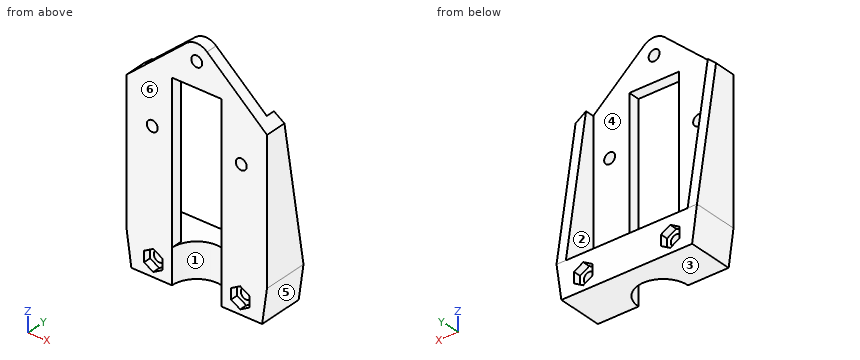
```python
from build123d import *

# Parameters (mm, degrees)
BOSS_EXTRUDE3_DEPTH              = 14.5
SKETCH8_R                        = 7.935
CUT_EXTRUDE3_DEPTH               = 88
CUT_EXTRUDE9_DEPTH               = 2.4
F_39_0_13779528_DIAMETER_HOLE1_D = 3.500000112
CUT_EXTRUDE10_DEPTH              = 22.4
CUT_EXTRUDE11_DEPTH              = 2.4
BOSS_EXTRUDE7_DEPTH              = 3.625
F_39_0_13779528_DIAMETER_HOLE2_D = 3.500000112
BOSS_EXTRUDE10_DEPTH             = 3
BOSS_EXTRUDE11_DEPTH             = 3
CUT_EXTRUDE14_DEPTH              = 13
CUT_EXTRUDE15_DEPTH              = 13
FILLET1_R                        = 5


with BuildPart() as part:
    # Sketch6 → Boss-Extrude3 (new body)
    with BuildSketch(Plane(origin=(0, 0, 0), x_dir=(1, 0, 0), z_dir=(0, 1, 0))):
        Polygon((-16.836914056, 5.783353512), (13.163085944, 5.783353512), (20.663085944, -47.581919406), (-24.336914056, -47.581919406), align=None)
    extrude(amount=BOSS_EXTRUDE3_DEPTH)

    # Sketch8 → Cut-Extrude3 (cut)
    with BuildSketch(Plane.XY.offset(47.581919406)):
        with Locations((-1.836914056, 0)):
            Circle(SKETCH8_R)
    extrude(amount=-CUT_EXTRUDE3_DEPTH, mode=Mode.SUBTRACT)

    # Sketch18 → Cut-Extrude9 (cut)
    with BuildSketch(Plane(origin=(0, 14.5, 0), x_dir=(1, 0, 0), z_dir=(0, 1, 0))):
        Polygon((-15.771819769, -44.868285994), (-12.821819769, -43.1651027), (-12.821819769, -39.758736112), (-15.771819769, -38.055552818), (-18.721819769, -39.758736112), (-18.721819769, -43.1651027), align=None)
        Polygon((12.097991657, -44.868285994), (15.047991657, -43.1651027), (15.047991657, -39.758736112), (12.097991657, -38.055552818), (9.147991657, -39.758736112), (9.147991657, -43.1651027), align=None)
        Polygon((11.389331688, -26.016021021), (14.389331688, -24.283970214), (14.389331688, -20.819868599), (11.389331688, -19.087817791), (8.389331688, -20.819868599), (8.389331688, -24.283970214), align=None)
        Polygon((-15.0631598, -26.016021021), (-12.0631598, -24.283970214), (-12.0631598, -20.819868599), (-15.0631598, -19.087817791), (-18.0631598, -20.819868599), (-18.0631598, -24.283970214), align=None)
    extrude(amount=-CUT_EXTRUDE9_DEPTH, mode=Mode.SUBTRACT)

    # #39 (0.13779528) Diameter Hole1 (through all)
    with Locations(Plane(origin=(-15.0631598, 14.5, 22.551919406), x_dir=(0, 0, 1), z_dir=(0, 1, 0))):
        with Locations((0, 0), (0, 26.452491488), (18.91, -0.708659969), (18.91, 27.161151457)):
            Hole(F_39_0_13779528_DIAMETER_HOLE1_D / 2)

    # Sketch22 → Cut-Extrude10 (cut)
    with BuildSketch(Plane(origin=(0, 14.5, 0), x_dir=(1, 0, 0), z_dir=(0, 1, 0))):
        Polygon((-22.781301734, -36.51316259), (19.107473622, -36.51316259), (13.163085944, 5.783353512), (-16.836914056, 5.783353512), align=None)
    extrude(amount=-CUT_EXTRUDE10_DEPTH, mode=Mode.SUBTRACT)

    # Sketch24 → Cut-Extrude11 (cut)
    with BuildSketch(Plane.XZ):
        Polygon((-15.771819769, 38.055552818), (-12.821819769, 39.758736112), (-12.821819769, 43.1651027), (-15.771819769, 44.868285994), (-18.721819769, 43.1651027), (-18.721819769, 39.758736112), align=None)
        Polygon((12.097991657, 38.055552818), (15.047991657, 39.758736112), (15.047991657, 43.1651027), (12.097991657, 44.868285994), (9.147991657, 43.1651027), (9.147991657, 39.758736112), align=None)
    extrude(amount=-CUT_EXTRUDE11_DEPTH, mode=Mode.SUBTRACT)

    # Sketch27 → Boss-Extrude7 (add)
    with BuildSketch(Plane(origin=(0, 0, 0), x_dir=(1, 0, 0), z_dir=(0, 1, 0))):
        Polygon((6.098085944, -47.581919406), (20.663085944, -47.581919406), (20.663085944, -112.581919406), (-9.771914056, -112.581919406), (-24.336914056, -112.581919406), (-24.336914056, -47.581919406), (-9.771914056, -47.581919406), (-9.771914056, -97.661919406), (6.098085944, -97.661919406), align=None)
    extrude(amount=BOSS_EXTRUDE7_DEPTH)

    # #39 (0.13779528) Diameter Hole2 (through all)
    with Locations(Plane(origin=(-16.086914056, 3.625, 80.900195398), x_dir=(0, 0, 1), z_dir=(0, 1, 0))):
        with Locations((0, 0), (24.681724008, 14.25), (0, 28.5)):
            Hole(F_39_0_13779528_DIAMETER_HOLE2_D / 2)

    # Sketch39 → Boss-Extrude10 (add)
    with BuildSketch(Plane(origin=(20.663085944, 0, 0), x_dir=(0, 0, -1), z_dir=(1, 0, 0))):
        Polygon((-47.581919406, 14.5), (-112.581919406, 3.625), (-47.581919406, 3.625), align=None)
    extrude(amount=-BOSS_EXTRUDE10_DEPTH)

    # Sketch40 → Boss-Extrude11 (add)
    with BuildSketch(Plane.ZY.offset(24.336914056)):
        Polygon((47.581919406, 14.5), (112.581919406, 3.625), (47.581919406, 3.625), align=None)
    extrude(amount=-BOSS_EXTRUDE11_DEPTH)

    # Sketch43 → Cut-Extrude14 (cut)
    with BuildSketch(Plane.XZ):
        Polygon((-1.836914056, 112.581919406), (-24.336914056, 112.581919406), (-24.336914056, 92.810231668), align=None)
    extrude(amount=-CUT_EXTRUDE14_DEPTH, mode=Mode.SUBTRACT)

    # Sketch44 → Cut-Extrude15 (cut)
    with BuildSketch(Plane.XZ):
        Polygon((20.663085944, 92.810231668), (20.663085944, 112.581919406), (-1.836914056, 112.581919406), align=None)
    extrude(amount=-CUT_EXTRUDE15_DEPTH, mode=Mode.SUBTRACT)

    # Fillet1
    fillet1_edges = [part.edges().sort_by_distance(p)[0] for p in [
        (-1.836914056, 1.8125, 112.581919406),
    ]]
    fillet(fillet1_edges, radius=FILLET1_R)


solid = part.part
```
Geometry: final body of the model. Coordinates: model frame, mm. Face numbers are marked on the shaded views. A direction names the side the tool comes from. Round coordinates to 2 decimals unless told otherwise and drop trailing zeros. Write each loop counter-clockwise with the first axis right and the second up, starting at its lowest first coordinate (ties: lowest second). Pieces come first, ordered by that corner, then holes.
Item 1: Pin query (flat end, axial travel): P1, Ø1.1, axis at x = -2, y = 2, coming from the -Z side; P2, Ø1.8, axis at x = 11, z = 41.5, coming from the -Y side; P3, Ø1.5, axis at x = 7.5, y = 7.5, coming from the +Z side. Return the tip coordinate at first contact, or that it passes through.
Item 2: Section query B-B (y = 9.75). Return loops of the section in (x, z), plus the area to 3 significant figures.
Item 3: Section query A-A (z = 78). Return loops of the section in (x, y) (3 decimals).
Item 4: Material intervals for L1, parallel to Z at x = -16, y = 2; L2, parallel to X at y = 5.75, z = 53.5; L3, parallel to X at y = 2.75, z = 71.5, sorted ascending.
Item 5: Set-up query: the marked faces 1, 2 and 3. Return all of +Z, -Z, +X, -X, +Y, -Y with unobstructed straight access to the full face (end or side cutting, diameter ignored); none if empty.
Item 6: Mould query, pull axis X, two halves, no side actions, for the marked faces 4, 5 and 6. Classes: +X half, -X half, draft (parallel to the pull), parting line (faces both ways), or undercut.
Item 7: Section query D-D (z = 59). Return loops of the section in (x, y) (3 decimals).
Item 8: Section query C-C (x = -7). Return loops of the section in (y, z) (1 decimal).
Completed:
1. P1: stops at z = 97.66
1. P2: stops at y = 2.4
1. P3: stops at z = 47.58
2. outline: (-24.34, 47.58) - (-22.78, 36.51) - (19.11, 36.51) - (20.66, 47.58) - (20.66, 75.97) - (17.66, 75.97) - (17.66, 47.58) - (-21.34, 47.58) - (-21.34, 75.97) - (-24.34, 75.97) - close; hole circle Ø3.5 at (-15.77, 41.46); hole circle Ø3.5 at (12.1, 41.46)
2. area: 632 mm2
3. outline: (-24.337, 0) - (-9.772, 0) - (-9.772, 3.625) - (-21.337, 3.625) - (-21.337, 9.411) - (-24.337, 9.411) - close; (6.098, 0) - (20.663, 0) - (20.663, 9.411) - (17.663, 9.411) - (17.663, 3.625) - (6.098, 3.625) - close
4. L1: z = 36.51 to 38.19, 44.74 to 79.15, 82.65 to 100.14
4. L2: x = -24.34 to -21.34, 17.66 to 20.66
4. L3: x = -24.34 to -9.77, 6.1 to 20.66
5. face 1: -Z, -Y
5. face 2: +Z, +Y
5. face 3: -Z, +X, -X, +Y, -Y
6. face 4: undercut
6. face 5: +X half
6. face 6: draft
7. outline: (-24.337, 0) - (-9.772, 0) - (-9.772, 3.625) - (-21.337, 3.625) - (-21.337, 12.59) - (-24.337, 12.59) - close; (6.098, 0) - (20.663, 0) - (20.663, 12.59) - (17.663, 12.59) - (17.663, 3.625) - (6.098, 3.625) - close
8. outline: (0, 97.7) - (3.6, 97.7) - (3.6, 108) - (0, 108) - close; (6, 36.5) - (14.5, 36.5) - (14.5, 47.6) - (6, 47.6) - close
